```python
from build123d import *

# Parameters (mm, degrees)
BOSS_EXTRUDE1_DEPTH = 1219.2
CUT_EXTRUDE1_DEPTH  = 134.35


with BuildPart() as part:
    # Sketch2 → Boss-Extrude1 (new body)
    with BuildSketch(Plane.XY):
        with BuildLine():
            Line((0, 0), (0, 31.75))
            Line((0, 31.75), (79.378619653, 133.35))
            Line((79.378619653, 133.35), (101.6, 133.35))
            Line((101.6, 133.35), (101.6, 114.3))
            ThreePointArc((101.6, 114.3), (74.403120681, 104.480352771), (58.99918365, 80.009667445))
            ThreePointArc((58.99918365, 80.009667445), (52.895666714, 56.49803793), (37.615267176, 37.615267176))
            Line((37.615267176, 37.615267176), (37.615267176, 28.090267176))
            ThreePointArc((37.615267176, 28.090267176), (17.75244877, 19.862818405), (9.525, 0))
            Line((9.525, 0), (0, 0))
        make_face()
    extrude(amount=BOSS_EXTRUDE1_DEPTH)

    # Sketch3 → Cut-Extrude1 (cut, through all)
    with BuildSketch(Plane(origin=(0, 133.35, 0), x_dir=(1, 0, 0), z_dir=(0, 1, 0))):
        Polygon((101.6, 0), (0, 0), (0, -101.6), align=None)
        Polygon((101.6, -1219.2), (0, -1219.2), (0, -1117.6), align=None)
    extrude(amount=-CUT_EXTRUDE1_DEPTH, mode=Mode.SUBTRACT)

    # Mirror4: part across plane


with BuildPart() as part_1:
    add(part.part)
    add(part.part.mirror(Plane(origin=(0, 0, 1117.6), x_dir=(0.707106781, 0, 0.707106781), z_dir=(0.707106781, 0, -0.707106781))))

    # Mirror5: part across plane


with BuildPart() as part_2:
    add(part_1.part)
    add(part_1.part.mirror(Plane(origin=(-1016, 0, 1117.6), x_dir=(-0.707106781, 0, 0.707106781), z_dir=(0.707106781, 0, 0.707106781))))


solid = part_2.part
```
Can you work these out from the model? Positions are in its coordinate system, mm. A direction names the side the tool comes from. Coordinates: 2 decimals unless noted, no trailing zeros. Order: outer loops, then holes, each group sorted by start corner. A loop starts at its lowest first (then second) coordinate and runs counter-clockwise, first axis right, second up.
1. I'm going to push flat-ended pins straight in: pin 1 (7.5 mm diameter, centred on x = -435.5, y = 34, fed in from -Z); pin 2 (9.5 mm diameter, centred on x = -417.5, y = 17, fed in from -Z); pin 3 (10.5 mm diameter, centred on x = -480, y = 31, fed in from +Z). Where does each tip first touch, or does it pass through?
2. Thinking about a two-plate mould opening in Z: for faces 4 (the face through (-499.47, 104.74, 26.87)), 5 (the face through (-516.53, 104.74, 1192.33)), 6 (the face through (-515, 16, 1117.6)), which applies, +Z half, -Z half, draft (parallel to the pull), parting line (faces both ways), or undercut?
3. If we section it at C-C (y = 95.5): Please give me the cut outline in (x, z).
4. I need wall thicknesses on line 1 (X direction, y = 119.5, z = 488); line 2 (Z direction, x = -271, y = 126); line 3 (X direction, y = 53, z = 108). Which ranges of each line are inside material? Lowest first, please.
5. If we section it at A-A (z = 487): Please give me the cut outline in (x, y) (3 decimals), then the cut area to 3 significant figures.
6. For faces 1 (the face through (-1016, 16, 617)), 2 (the face through (-500.062, 56.804, 48.551)), 3 (the face through (-516.223, 81.839, 1156.734)), which set-ups out of +Z, -Z, +X, -X, +Y, -Y let a thin tool reach every point of the face, with its end or its side?
7. If we section it at B-B (x = -263): Please give me the cut outline in (y, z) (3 decimals), then the cut area to 3 significant figures.
Entries:
1. pin 1: stops at z = 63.82
1. pin 2: stops at z = 81.76
1. pin 3: stops at z = 1155.22
2. face 4: -Z half
2. face 5: +Z half
2. face 6: undercut
3. outline: (-1081.97, 35.63) - (65.97, 35.63) - (65.97, 1183.57) - (-1081.97, 1183.57) - close; hole (-1065.81, 51.79) - (49.81, 51.79) - (49.81, 1167.41) - (-1065.81, 1167.41) - close
4. line 1: x = -1117.6 to -1084.56, 68.56 to 101.6
4. line 2: z = 0 to 27.96, 1191.24 to 1219.2
4. line 3: x = -1066.98 to -1032.6, 16.6 to 50.98
5. outline: (-1117.6, 114.3) arc R44.455 cw to (-1074.999, 80.01) arc R57.408 ccw to (-1053.615, 37.615) - (-1053.615, 28.09) arc R28.09 cw to (-1025.525, 0) - (-1016, 0) - (-1016, 31.75) - (-1095.379, 133.35) - (-1117.6, 133.35) - close; (0, 0) - (9.525, 0) arc R28.09 cw to (37.615, 28.09) - (37.615, 37.615) arc R57.408 ccw to (58.999, 80.01) arc R44.455 cw to (101.6, 114.3) - (101.6, 133.35) - (79.379, 133.35) - (0, 31.75) - close
5. area: 6,630 mm2
6. face 1: +Y, -Y
6. face 2: -Z, +X, -X, -Y
6. face 3: +Y
7. outline: (0, 92.075) arc R28.09 cw to (28.09, 63.985) - (37.615, 63.985) arc R57.408 ccw to (80.01, 42.601) arc R44.455 cw to (114.3, 0) - (133.35, 0) - (133.35, 22.221) - (31.75, 101.6) - (0, 101.6) - close; (0, 1117.6) - (31.75, 1117.6) - (133.35, 1196.979) - (133.35, 1219.2) - (114.3, 1219.2) arc R44.455 cw to (80.01, 1176.599) arc R57.408 ccw to (37.615, 1155.215) - (28.09, 1155.215) arc R28.09 cw to (0, 1127.125) - close
7. area: 6,630 mm2
